Input: part model. Units: mm. Frame: model coordinates. A direction names the side the tool comes from. Round coordinates to 2 decimals unless told otherwise and drop trailing zeros. Loops run counter-clockwise (first coordinate to the right, second up) from the corner with the lowest first, then second, coordinate; pieces in that order, holes last. Notation, with made-up numbers: (53.25, 45.25) - (69.25, 45.25) arc R14 cw to (69.25, 56.25) - close; hole circle Ø8 at (82, -2.5). An arc over 180 degrees is marked (long way). Write each question's results on one line, items separated by ' | '.
Autodesk Inventor part; units mm, degrees
ref_plane "YZ Plane" through (0, 0, 0) normal (1, 0, 0) x (0, 1, 0)
ref_plane "XZ Plane" through (0, 0, 0) normal (0, 1, 0) x (-1, 0, 0)
ref_plane "XY Plane" through (0, 0, 0) normal (0, 0, 1) x (1, 0, 0)
sketch "Sketch1" plane through (0, 0, 0) normal (0, 1, 0) x (-1, 0, 0)
  circle A0 centre (0, 0) radius 3.5
  dimension "d0" = 7
extrude "Extrusion1" add sketch "Sketch1" against normal blind 4
sketch "Sketch2" plane through (0, -4, 0) normal (0, -1, 0) x (1, 0, 0)
  circle A0 centre (0, 0) radius 2
  dimension "d3" = 4
extrude "Extrusion2" add sketch "Sketch2" along normal blind 20
sketch "Sketch3" plane through (0, 0, 0) normal (0, 1, 0) x (1, 0, 0)
  circle A0 centre (0, 0) radius 2 construction
  line L0 (1.7321, 0) -> (0.866, -1.5)
  line L1 (0.866, -1.5) -> (-0.866, -1.5)
  line L2 (-0.866, -1.5) -> (-1.7321, 0)
  line L3 (-1.7321, 0) -> (-0.866, 1.5)
  line L4 (-0.866, 1.5) -> (0.866, 1.5)
  line L5 (0.866, 1.5) -> (1.7321, 0)
  dimension "d8" = 3
extrude "Extrusion3" cut sketch "Sketch3" against normal blind 1.5
chamfer "Chamfer1" distance 0.25 angle 45 1 edges at (-2, -24, 0)
fillet "Fillet1" radius 0.25 2 edges at (3.5, 0, 0) (3.5, -4, 0)
chamfer "Chamfer2" distance 0.1 angle 45 6 edges at (0, 0, -1.5) (1.299, 0, -0.75) (1.299, 0, 0.75) (0, 0, 1.5) (-1.299, 0, 0.75) (-1.299, 0, -0.75)
thread "Thread2"
properties part number "M4-20" material "Steel, Carbon"
1. Contact query for flat-ended pins moving along their axis: pin 1 (1 mm diameter, centred on y = -15.5, z = -1.5, fed in from -X); pin 2 (0.7 mm diameter, centred on x = 0.5, y = -0.5, fed in from -Z); pin 3 (1.5 mm diameter, centred on x = -1, y = -5, fed in from +Z). Output: stop coordinate, or through.
Answer:
pin 1: x = -1.73 | pin 2: z = -3.5 | pin 3: z = 1.98
2. Mould query, pull axis Z, two halves, no side actions, for faces 4 (the cylindrical face through (-3.233, -1.976, -1.341)), 5 (the flat face through (0, -24, 0)), 6 (the flat face through (0, -1.5, 0)). Classes: pulls with the +Z half, pulls with the -Z half, needs draft (parallel to the pull), parting line crosses it, or undercut.
Answer:
face 4: parting line crosses it | face 5: needs draft | face 6: undercut
3. Section query A-A, the plane x = 0. Output: boundary loops of the cut face in (y, z).
Answer:
outline: (-24, -1.75) - (-23.75, -2) - (-4, -2) - (-4, -3.25) arc R0.25 ccw to (-3.75, -3.5) - (-0.25, -3.5) arc R0.25 ccw to (0, -3.25) - (0, -1.6) - (-0.1, -1.5) - (-1.5, -1.5) - (-1.5, 1.5) - (-0.1, 1.5) - (0, 1.6) - (0, 3.25) arc R0.25 ccw to (-0.25, 3.5) - (-3.75, 3.5) arc R0.25 ccw to (-4, 3.25) - (-4, 2) - (-23.75, 2) - (-24, 1.75) - close
4. Line query: line 1 (Y direction, x = -1.25, z = -2); line 2 (Z direction, x = -1, y = -16.25); line 3 (Z direction, x = 0.5, y = -8.5). Output: solid intervals per line, ascending. Write a range as [from, to].
Answer:
line 1: [-4, 0] | line 2: [-1.73, 1.73] | line 3: [-1.94, 1.94]
5. Set-up query: faces 1 (the flat face through (-1, -4, -2)), 2 (the flat face through (-1.4, 0, -1.4)), 3 (the flat face through (-1.305, -0.79, -0.74)). Return all of +Z, -Z, +X, -X, +Y, -Y with unobstructed straight access to the full face (end or side cutting, diameter ignored); none if empty.
Answer:
face 1: -Y | face 2: +Z, -Z, +X, -X, +Y | face 3: +Y
6. Section query B-B, the plane y = -17.75. Output: boundary loops of the cut face in (x, z).
Answer:
outline: circle Ø4 at (0, 0)
